For this review, take the finished solid that the model builds, in its own axes (mm). Face numbers are marked on the shaded views. Give positions to 0.01 mm unless a question says otherwise; leave off trailing zeros. Loops run counter-clockwise (first coordinate to the right, second up) from the corner with the lowest first, then second, coordinate; pieces in that order, holes last. Notation, with made-up numbers: (-31.5, 26) - (-19.5, 26) arc R19 cw to (-19.5, 35) - close; hole circle Ø11 at (64, -15). An arc over 180 degrees is marked (long way). Put each result on its own line as item: value. Start each with the question number.
from build123d import *

# Parameters (mm, degrees)
SKETCH1_R           = 5.95
BOSS_EXTRUDE1_DEPTH = 8.8
SKETCH2_R           = 1
CUT_EXTRUDE1_DEPTH  = 2
CHAMFER1_SIZE       = 0.5
SKETCH3_R           = 0.25
BOSS_EXTRUDE2_DEPTH = 5


with BuildPart() as part:
    # Sketch1 → Boss-Extrude1 (new body)
    with BuildSketch(Plane(origin=(0, 0, 0), x_dir=(1, 0, 0), z_dir=(0, 1, 0))):
        with Locations(Location((0, 0, 0), (0, 0, 270))):
            Circle(SKETCH1_R)
    extrude(amount=BOSS_EXTRUDE1_DEPTH)

    # Sketch2 → Cut-Extrude1 (cut)
    with BuildSketch(Plane(origin=(0, 8.8, 0), x_dir=(1, 0, 0), z_dir=(0, 1, 0))):
        with Locations(Location((0, 0, 0), (0, 0, 270))):
            Circle(SKETCH2_R)
    extrude(amount=-CUT_EXTRUDE1_DEPTH, mode=Mode.SUBTRACT)

    # Chamfer1
    chamfer1_edges = [part.edges().sort_by_distance(p)[0] for p in [
        (0, 8.8, -5.95),
    ]]
    chamfer(chamfer1_edges, length=CHAMFER1_SIZE)

    # Sketch3 → Boss-Extrude2 (add)
    with BuildSketch(Plane.XZ):
        with Locations(Location((-3, 0, 0), (0, 0, 90))):
            Circle(SKETCH3_R)
    boss_extrude2 = extrude(amount=BOSS_EXTRUDE2_DEPTH)

    # Mirror1: Boss-Extrude2 across plane
    add(boss_extrude2.mirror(Plane(origin=(0, 0, 0), x_dir=(0, 0, 1), z_dir=(1, 0, 0))))


solid = part.part
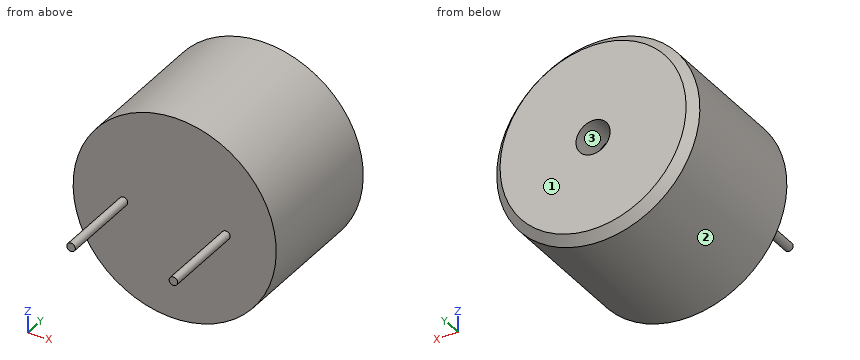
1) Take a section at C-C on y = 7.5. State the section outline as (x, z) points, and give its area (3 significant figures).
2) Mouldability with a two-part tool opening along X and no side actions: class the marked faces 1, 2 and 3 as released by +X, released by -X, zero draft, split by the parting line, or undercut.
3) Take a section at D-D on y = -1.75. State the section outline as (x, z) points, and give its area (3 significant figures).
4) Take a section at A-A on x = 0. State the section outline as (y, z) points.
5) Insertion check: P1, Ø2, axis at y = 3, z = 3.5, coming from the -X side. The pin has a flat end and moves straight along its axis. Give the tip position at first contact, or say it passes through.
6) Take a section at B-B on z = 0. State the section outline as (x, y) points.
7) Wall thickness on probe 1 along X at (y, z) = (7.95, 0); probe 2 along X at (y, z) = (-2.75, 0); probe 3 along Y at (x, z) = (1, -0.5): over which ranges is each line inside the solid? List them lowest first.
Answers follow:
1. outline: circle Ø11.9 at (0, 0); hole circle Ø2 at (0, 0)
1. area: 108 mm2
2. face 1: zero draft
2. face 2: split by the parting line
2. face 3: undercut
3. outline: circle Ø0.5 at (-3, 0); circle Ø0.5 at (3, 0)
3. area: 0.393 mm2
4. outline: (0, -5.95) - (8.3, -5.95) - (8.8, -5.45) - (8.8, -1) - (6.8, -1) - (6.8, 1) - (8.8, 1) - (8.8, 5.45) - (8.3, 5.95) - (0, 5.95) - close
5. P1: x = -5.4
6. outline: (-5.95, 0) - (-3.25, 0) - (-3.25, -5) - (-2.75, -5) - (-2.75, 0) - (2.75, 0) - (2.75, -5) - (3.25, -5) - (3.25, 0) - (5.95, 0) - (5.95, 8.3) - (5.45, 8.8) - (1, 8.8) - (1, 6.8) - (-1, 6.8) - (-1, 8.8) - (-5.45, 8.8) - (-5.95, 8.3) - close
7. probe 1: -5.95 to -1, 1 to 5.95
7. probe 2: -3.25 to -2.75, 2.75 to 3.25
7. probe 3: 0 to 8.8
